from build123d import *

# Parameters (mm, degrees)
SKETCH1_R           = 10
BOSS_EXTRUDE1_DEPTH = 10


with BuildPart() as part:
    # Sketch1 → Boss-Extrude1 (new body)
    with BuildSketch(Plane.XY):
        with BuildLine():
            ThreePointArc((-15, -75.267843328), (0, -90.267843328), (15, -75.267843328))
            add(Edge.make_bspline(
                [(15, 204.732156672), (4.423835308, 157.931962062), (15, -75.267843328)],
                knots=[0, 0, 0, 1, 1, 1], degree=2))
            ThreePointArc((15, 204.732156672), (0, 219.732156672), (-15, 204.732156672))
            add(Edge.make_bspline(
                [(-15, 204.732156672), (-6.422661748, 158.481211522), (-15, -75.267843328)],
                knots=[0, 0, 0, 1, 1, 1], degree=2))
        make_face()
        with Locations((0, -75.267843328)):
            Circle(SKETCH1_R, mode=Mode.SUBTRACT)
        with Locations((0, 204.732156672)):
            Circle(SKETCH1_R, mode=Mode.SUBTRACT)
    extrude(amount=BOSS_EXTRUDE1_DEPTH)


solid = part.part
Model file for the job. Use its own axes, mm. Give positions to 0.01 mm unless a question says otherwise; leave off trailing zeros. Loops run counter-clockwise (first coordinate to the right, second up) from the corner with the lowest first, then second, coordinate; pieces in that order, holes last.
Item 1: Mould opens along Y. For faces 1 (the face through (-2.17, -85.03, 4.93)), 2 (the face through (0, 67, 0)), 3 (the face through (0.33, 219.73, 4.93)) say: +Y half, -Y half, draft (parallel to the pull), parting line (faces both ways), or undercut.
Check values:
face 1: undercut
face 2: draft
face 3: +Y half
Item 2: Slice it at B-B (z = 2.25). Give the number of separate pieces and of enclosed holes in the cut face, plus the area to 3 significant figures.
Check values:
separate pieces: 1
enclosed holes: 2
area: 6,690 mm2
Item 3: Slice it at A-A (x = 0). Write the cut outline in (y, z), plus the area to 3 significant figures.
Check values:
outline: (-90.27, 0) - (-85.27, 0) - (-85.27, 10) - (-90.27, 10) - close; (-65.27, 0) - (194.73, 0) - (194.73, 10) - (-65.27, 10) - close; (214.73, 0) - (219.73, 0) - (219.73, 10) - (214.73, 10) - close
area: 2,700 mm2
Item 4: Drop flat-ended pins along their axis: P1, Ø4, axis at y = -43.5, z = 5, coming from the -X side; P2, Ø1.5, axis at x = 6.5, z = 7.5, coming from the +Y side; P3, Ø5, axis at x = 11.5, z = 4, coming from the -Y side. Give the stop position or say it passes through.
Check values:
P1: stops at x = -13.95
P2: stops at y = 218.59
P3: stops at y = -87.27
Item 5: Drill centre lines: line 1 along Y through (x, z) = (0, 3); line 2 along Y through (x, z) = (3, 7); line 3 along X through (y, z) = (-37, 9.5). Where is each one in solid material? Low to high.
Check values:
line 1: y = -90.27 to -85.27, -65.27 to 194.73, 214.73 to 219.73
line 2: y = -89.96 to -84.81, -65.73 to 195.19, 214.27 to 219.43
line 3: x = -13.67 to 13.36
